Autodesk Inventor part; units mm, degrees
ref_plane "YZ Plane" through (0, 0, 0) normal (1, 0, 0) x (0, 1, 0)
ref_plane "XZ Plane" through (0, 0, 0) normal (0, 1, 0) x (-1, 0, 0)
ref_plane "XY Plane" through (0, 0, 0) normal (0, 0, 1) x (1, 0, 0)
sketch "Schizzo1" plane through (0, 0, 0) normal (0, 1, 0) x (-1, 0, 0)
  circle A0 centre (0, 0) radius 15
  circle A1 centre (0, 0) radius 40
  dimension "d0" = 30
  dimension "d1" = 80
extrude "Estrusione1" add sketch "Schizzo1" against normal blind 34
sketch "Schizzo2" plane through (0, -34, 0) normal (0, -1, 0) x (1, 0, 0)
  circle A0 centre (0, 0) radius 15
  circle A1 centre (0, 0) radius 42.5
  dimension "d4" = 85
extrude "Estrusione2" add sketch "Schizzo2" against normal blind 34
sketch "Schizzo3" plane through (0, -34, 0) normal (0, -1, 0) x (1, 0, 0)
  circle A0 centre (0, 0) radius 34.885
  line L0 (0, 41.5801) -> (0, 0)
  line L1 (0, 0) -> (-42.3383, -3.7041)
  circle A1 centre (0, 0) radius 42.5
  line L2 (42.3383, -3.7041) -> (0, 0)
  point P0 (-34.7523, -3.0404)
  point P1 (34.7523, -3.0404)
  dimension "d7" = 69.77
  dimension "d8" = 95
  dimension "d9" = 95
hole "Foro1" at (-34.7523, -34, -3.0404) at (34.7523, -34, -3.0404) direction (0, 1, 0) diameter 11.4 depth 19.8 tip angle 118
sketch "Schizzo4" plane through (0, -34, 0) normal (0, -1, 0) x (1, 0, 0)
  circle A0 centre (0, 0) radius 34.885
  point P0 (0, 34.885)
  dimension "d17" = 69.77
hole "Foro2" at (0, -34, 34.885) direction (0, 1, 0) diameter 10.262 depth 34 tip angle 118
properties part number "forato" material "Ferro, Ghisa grigia ASTM A48 Grado 20"
Part model, mm, in its own coordinate system. A direction names the side the tool comes from. Round coordinates to 2 decimals unless told otherwise and drop trailing zeros. Loops run counter-clockwise (first coordinate to the right, second up) from the corner with the lowest first, then second, coordinate; pieces in that order, holes last.
Item 1: Drill centre lines: line 1 (Z direction, x = 0, y = -17); line 2 (Z direction, x = 3.5, y = -3); line 3 (Z direction, x = 11, y = -30). Where is each one in solid material? Low to high.
Item 2: Cut at D-D, the plane y = -17. Give the cut face in (x, z) (3 decimals), then the cut area to 3 significant figures.
Item 3: Cut at C-C, the plane x = -14. Give the cut face in (y, z).
Item 4: Mould opens along X. For faces 3 (the face through (1, -34, -18)), 4 (the face through (-33.92, -11.37, -3.57)), 5 (the face through (-33.727, -17.238, -25.861)) say: +X half, -X half, draft (parallel to the pull), parting line (faces both ways), or undercut.
Item 5: 3-axis set-ups, long thin cutter, end or side, ignore diameter. For faces 1 (the face through (40.317, -23.961, -1.805)), 2 (the face through (14.985, -16.762, 0.66)): which of +Z, -Z, +X, -X, +Y, -Y reach the whole face in a straight line?
Item 6: Drop flat-ended pins along their axis: P1, Ø5, axis at y = -22.5, z = 33.5, coming from the +X side; P2, Ø18, axis at x = 0, z = 0, coming from the +Y side; P3, Ø10, axis at y = -13, z = -8, coming from the +X side; P4, Ø10.5, axis at x = -34.75, z = -3.04, coming from the -Y side. Give the stop position or say it passes through.
Item 7: Cut at B-B, the plane z = 4.5. Give the cut face in (x, y), then the cut area to 3 significant figures.
Item 8: Cut at A-A, the plane x = 0. Give the cut face in (y, z).
A:
1. line 1: z = -42.5 to -15, 15 to 29.75, 40.02 to 42.5
1. line 2: z = -42.36 to -14.59, 14.59 to 31.13, 38.64 to 42.36
1. line 3: z = -41.05 to -10.2, 10.2 to 41.05
2. outline: circle Ø85 at (0, 0); hole circle Ø11.4 at (-34.752, -3.04); hole circle Ø30 at (0, 0); hole circle Ø10.262 at (0, 34.885); hole circle Ø11.4 at (34.752, -3.04)
2. area: 4,680 mm2
3. outline: (-34, -40.13) - (0, -40.13) - (0, -5.39) - (-34, -5.39) - close; (-34, 5.39) - (0, 5.39) - (0, 40.13) - (-34, 40.13) - close
4. face 3: draft
4. face 4: undercut
4. face 5: parting line
5. face 1: -Y
5. face 2: +Y, -Y
6. P1: stops at x = 29.07
6. P2: passes through
6. P3: stops at x = 42.39
6. P4: stops at y = -13.93
7. outline: (-42.26, -34) - (-14.31, -34) - (-14.31, 0) - (-42.26, 0) - close; (14.31, -34) - (42.26, -34) - (42.26, 0) - (14.31, 0) - close
7. area: 1,900 mm2
8. outline: (-34, -42.5) - (0, -42.5) - (0, -15) - (-34, -15) - close; (-34, 15) - (0, 15) - (0, 29.75) - (-34, 29.75) - close; (-34, 40.02) - (0, 40.02) - (0, 42.5) - (-34, 42.5) - close
